Autodesk Inventor part; units mm, degrees
ref_plane "YZ Plane" through (0, 0, 0) normal (1, 0, 0) x (0, 1, 0)
ref_plane "XZ Plane" through (0, 0, 0) normal (0, 1, 0) x (-1, 0, 0)
ref_plane "XY Plane" through (0, 0, 0) normal (0, 0, 1) x (1, 0, 0)
sketch "Skizze3" plane through (0, 0, 0) normal (0, 0, 1) x (1, 0, 0)
  line L0 (0, 0) -> (5.4656, 0)
  line L1 (5.4656, 0) -> (9.75, 3)
  line L2 (9.75, 3) -> (9.75, 5)
  line L3 (9.75, 5) -> (0, 5)
  line L4 (0, 6) -> (0, -1) construction
  line L5 (0, 0) -> (-5.4656, 0)
  line L6 (-5.4656, 0) -> (-9.75, 3)
  line L7 (-9.75, 3) -> (-9.75, 5)
  line L8 (-9.75, 5) -> (0, 5)
  dimension "d6" = 9.75
  dimension "d8" = 5
  dimension "d9" = 3
  dimension "d10" = 145
extrude "Extrusion2" add sketch "Skizze3" along normal mid plane 8
sketch "Skizze4" plane through (-9.75, 5, 4) normal (0, 1, 0) x (1, 0, 0)
  line L0 (0, 8) -> (0, 0)
  line L1 (19.5, 0) -> (0, 0)
  line L2 (19.5, 8) -> (19.5, 0)
  line L3 (0, 8) -> (19.5, 8)
  circle A0 centre (9.75, 4) radius 1.5
  line L4 (5.75, 8) -> (13.75, 8)
  line L5 (13.75, 8) -> (13.75, 0)
  line L6 (13.75, 0) -> (5.75, 0)
  line L7 (5.75, 0) -> (5.75, 8)
  line L8 (5.75, 8) -> (13.75, 0) construction
  line L9 (13.75, 8) -> (5.75, 0) construction
  line L10 (0, 8) -> (19.5, 8)
  arc A1 (9.75, 8) -> (5.75, 4) centre (9.75, 4) ccw
  arc A2 (9.75, 0) -> (13.75, 4) centre (9.75, 4) ccw
  point P0 (9.75, 0)
  dimension "d13" = 3
  dimension "d14" = 8
  dimension "d15" = 8
extrude "Extrusion3" add sketch "Skizze4" along normal blind 3 and the other way blind 5 separate body contours L7 A1 L3 L5 A2 L1
sketch "Skizze5" plane through (9.75, 3, 4) normal (1, 0, 0) x (0, 0, -1)
  line L0 (8, 2) -> (0, 2)
  line L1 (0, 0) -> (0, 2)
  line L2 (8, 0) -> (0, 0)
  line L3 (8, 2) -> (8, 0)
  line L4 (0, 0) -> (0, 2)
  line L5 (0, 2) -> (0.495, 1.505)
  line L6 (0.495, 1.505) -> (0.9899, 2)
  line L7 (8, 2) -> (0, 2)
  line L8 (1.15, 2) -> (1.645, 1.505)
  line L9 (1.645, 1.505) -> (2.1399, 2)
  line L10 (2.3, 2) -> (2.795, 1.505)
  line L11 (2.795, 1.505) -> (3.2899, 2)
  line L12 (3.45, 2) -> (3.945, 1.505)
  line L13 (3.945, 1.505) -> (4.4399, 2)
  line L14 (4.6, 2) -> (5.095, 1.505)
  line L15 (5.095, 1.505) -> (5.5899, 2)
  line L16 (5.75, 2) -> (6.245, 1.505)
  line L17 (6.245, 1.505) -> (6.7399, 2)
  line L18 (6.9, 2) -> (7.395, 1.505)
  line L19 (7.395, 1.505) -> (7.8899, 2)
  point P0 (4, -3)
  dimension "d21" = 0.7
  dimension "d24" = 1.15
extrude "Extrusion4" cut sketch "Skizze5" against normal up to surface (19.5 mm away) contours L19 L18 L0 | L17 L16 L0 | L0 L6 L5 | L15 L14 L0 | L0 L9 L8 | L13 L12 L0 | L0 L11 L10 bodies 1
extrude "Extrusion5" cut sketch "Skizze4" against normal blind 10 contours A0 bodies 1
chamfer "Fase2" distance 1 angle 45 1 edges at (-1.5, 8, 0)
combine bodies "Kombinieren1" operation type add bodies to combine 1 2
fillet "Rundung1" radius 2 2 edges at (9.75, 4, 4) (-9.75, 4, -4)
properties part number "T-NUT - DropIn 4040 SERIES - M3"
The model under review builds one solid part; all positions refer to its coordinate system, in mm. Give positions to 0.01 mm unless a question says otherwise; leave off trailing zeros. Write each loop counter-clockwise with the first axis right and the second up, starting at its lowest first coordinate (ties: lowest second). Pieces come first, ordered by that corner, then holes.
(1) Consider section B-B, the plane x = -7.5. Give the boundary of the cut face in (y, z) (3 decimals).
(2) To check wall thickness, follow L1, parallel to Z at x = 0, y = 3.25; L2, parallel to X at y = 4, z = 0. State the ranges of each line that lie inside material, in increasing order.
(3) The part is to be moulded in two halves that separate along Z. For faces 1 (the cylindrical face through (-8.88, 3.7, -3.65)), 2 (the cylindrical face through (-1.5, 3.55, -0.07)), 3 (the cylindrical face through (8.88, 3.7, 3.65)), 4 (the flat face through (-7.58, 1.48, -0.06)), say which applies: released by +Z, released by -Z, zero draft, split by the parting line, or undercut.
(4) For P1, Ø1, axis at x = 5.5, z = -1.5, coming from the +Y side; P2, Ø4, axis at y = 5, z = -2, coming from the -X side; P3, Ø1, axis at x = 2.5, y = 6.5, coming from the +Z side, all flat-tipped, find the tip position at first contact; note any pin that passes through.
(5) Consider section A-A, the plane x = -4.5. Give the boundary of the cut face in (y, z) (3 decimals).
Returned:
1. outline: (1.425, -4) - (5, -4) - (5, -3.89) - (4.505, -3.395) - (5, -2.9) - (5, -2.74) - (4.505, -2.245) - (5, -1.75) - (5, -1.59) - (4.505, -1.095) - (5, -0.6) - (5, -0.44) - (4.505, 0.055) - (5, 0.55) - (5, 0.71) - (4.505, 1.205) - (5, 1.7) - (5, 1.86) - (4.505, 2.355) - (5, 2.85) - (5, 3.01) - (4.505, 3.505) - (5, 4) - (1.425, 4) - close
2. L1: z = -4 to -1.5, 1.5 to 4
2. L2: x = -9.75 to -1.5, 1.5 to 9.75
3. face 1: released by -Z
3. face 2: undercut
3. face 3: released by +Z
3. face 4: zero draft
4. P1: stops at y = 5
4. P2: stops at x = -9.75
4. P3: stops at z = 3.46
5. outline: (0, -4) - (5, -4) - (5, -3.89) - (4.505, -3.395) - (5, -2.9) - (5, -2.74) - (4.505, -2.245) - (5, -1.75) - (5, -1.59) - (4.505, -1.095) - (5, -0.6) - (5, -0.44) - (4.505, 0.055) - (5, 0.55) - (5, 0.71) - (4.505, 1.205) - (5, 1.7) - (5, 1.86) - (4.505, 2.355) - (5, 2.85) - (5, 3.01) - (4.505, 3.505) - (5, 4) - (0, 4) - close
